Autodesk Inventor part; units mm, degrees
ref_plane "YZ Plane" through (0, 0, 0) normal (1, 0, 0) x (0, 1, 0)
ref_plane "XZ Plane" through (0, 0, 0) normal (0, 1, 0) x (-1, 0, 0)
ref_plane "XY Plane" through (0, 0, 0) normal (0, 0, 1) x (1, 0, 0)
sketch "Sketch1" plane through (0, 0, 0) normal (0, 0, 1) x (1, 0, 0)
  line L0 (-177.8, 0) -> (0, 0)
  line L1 (0, 0) -> (0, 127)
  line L2 (-169.9735, 254) -> (-355.6, 254)
  line L3 (-355.6, 254) -> (-355.6, 127)
  line L4 (-355.6, 127) -> (-228.6, 127)
  line L5 (-228.6, 127) -> (-177.8, 0)
  line L6 (-169.9735, 254) -> (-119.1735, 127)
  line L7 (-119.1735, 127) -> (0, 127)
  dimension "d8" = 127
  dimension "brkt_ht" = 254
  dimension "brkt_width" = 355.6
  dimension "d11" = 127
  dimension "d12" = 101.6
  dimension "d13" = 111.801
  dimension "d15" = 177.8
extrude "Extrusion1" add sketch "Sketch1" along normal blind 12.7
fillet "Fillet1" radius 25.4 2 edges at (-228.6, 127, 6.35) (-119.1735, 127, 6.35)
sketch "Sketch4" plane through (0, 0, 12.7) normal (0, 0, 1) x (1, 0, 0)
  line L0 (-25.4, 101.6) -> (-82.55, 101.6) construction
  line L1 (-82.55, 101.6) -> (-82.55, 25.4) construction
  line L2 (-82.55, 25.4) -> (-25.4, 25.4) construction
  line L3 (-25.4, 25.4) -> (-25.4, 101.6) construction
  line L4 (0, 0) -> (0, 127) construction
  line L5 (0, 127) -> (-101.9768, 127) construction
  point P0 (-25.4, 63.5)
  point P1 (0, 63.5)
  dimension "d19" = 25.4
  dimension "d20" = 25.4
  dimension "d21" = 57.15
hole "Hole1" at (-25.4, 101.6, 12.7) at (-82.55, 101.6, 12.7) at (-82.55, 25.4, 12.7) at (-25.4, 25.4, 12.7) direction (0, 0, -1) diameter 13.4874 end through all
properties part number "884702-01"
Geometry: final body of the model. Coordinates: model frame, mm. A direction names the side the tool comes from. Coordinates: 2 decimals unless noted, no trailing zeros. Order: outer loops, then holes, each group sorted by start corner. A loop starts at its lowest first (then second) coordinate and runs counter-clockwise, first axis right, second up. Notation, with made-up numbers: (54.25, 44.5) - (93.25, 44.5) arc R18 cw to (93.25, 55.5) - close; hole circle Ø11 at (21.25, 70.25). An arc over 180 degrees is marked (long way). Write each question's results on one line, items separated by ' | '.
(1) Section query B-B, the plane z = 2. Return the cut outline in (x, y), plus the area to 3 significant figures.
Values found:
outline: (-355.6, 127) - (-245.8, 127) arc R25.4 cw to (-222.21, 111.03) - (-177.8, 0) - (0, 0) - (0, 127) - (-101.98, 127) arc R25.4 cw to (-125.56, 142.97) - (-169.97, 254) - (-355.6, 254) - close; hole circle Ø13.49 at (-82.55, 25.4); hole circle Ø13.49 at (-82.55, 101.6); hole circle Ø13.49 at (-25.4, 25.4); hole circle Ø13.49 at (-25.4, 101.6) | area: 52,100 mm²
(2) Section query A-A, the plane y = 101.6. Return the cut outline in (x, z), plus the area to 3 significant figures.
Values found:
outline: (-218.44, 0) - (-89.29, 0) - (-89.29, 12.7) - (-218.44, 12.7) - close; (-75.81, 0) - (-32.14, 0) - (-32.14, 12.7) - (-75.81, 12.7) - close; (-18.66, 0) - (0, 0) - (0, 12.7) - (-18.66, 12.7) - close | area: 2,430 mm²
(3) Line query: line 1 (Y direction, x = -82.55, z = 5); line 2 (X direction, y = 25.4, z = 5.25); line 3 (X direction, y = 101.6, z = 9.75). Output: solid intervals per line, ascending. Write a range as [from, to].
Values found:
line 1: y = [0, 18.66], [32.14, 94.86], [108.34, 127] | line 2: x = [-187.96, -89.29], [-75.81, -32.14], [-18.66, 0] | line 3: x = [-218.44, -89.29], [-75.81, -32.14], [-18.66, 0]
(4) Set-up query: faces 1 (the face through (-25.697, 108.337, 6.261)), 2 (the face through (-52, 127, 6)), 3 (the face through (-301, 127, 6)). Return all of +Z, -Z, +X, -X, +Y, -Y with unobstructed straight access to the full face (end or side cutting, diameter ignored); none if empty.
Values found:
face 1: +Z, -Z | face 2: +Z, -Z, +X, +Y | face 3: +Z, -Z, -X, -Y
(5) Mould query, pull axis Y, two halves, no side actions, for faces 4 (the face through (-116.392, 131.486, 6.439)), 5 (the face through (-355.6, 191, 6)), 6 (the face through (-76.567, 22.288, 6.261)), 7 (the face through (-78.447, 106.952, 6.261)). Classes: +Y half, -Y half, draft (parallel to the pull), parting line (faces both ways), or undercut.
Values found:
face 4: +Y half | face 5: draft | face 6: undercut | face 7: undercut
(6) First-contact query: pin 1 Ø4 at (y, z) = (44.5, 2) entering from -X; pin 2 Ø15.5 at (x, y) = (-82.55, 101.6) entering from +Z; pin 3 Ø4 at (y, z) = (79.5, 4.5) entering from -X; pin 4 Ø4 at (x, z) = (-66.5, 8) entering from +Y. Flat tips, straight axial feed; report the tip coordinate or a pass-through.
Values found:
pin 1: stops at x = -196.4 | pin 2: stops at z = 12.7 | pin 3: stops at x = -210.4 | pin 4: stops at y = 127
(7) Section query C-C, the plane x = -82.55. Return the cut outline in (y, z), plus the area to 3 significant figures.
Values found:
outline: (0, 0) - (18.66, 0) - (18.66, 12.7) - (0, 12.7) - close; (32.14, 0) - (94.86, 0) - (94.86, 12.7) - (32.14, 12.7) - close; (108.34, 0) - (127, 0) - (127, 12.7) - (108.34, 12.7) - close | area: 1,270 mm²
(8) Section query D-D, the plane x = -279. Return the cut outline in (y, z), plus the area to 3 significant figures.
Values found:
outline: (127, 0) - (254, 0) - (254, 12.7) - (127, 12.7) - close | area: 1,610 mm²
